Here's how the part is built. I have some questions about the finished solid (model axes, mm). Face numbers are marked on the shaded views. Round coordinates to 2 decimals unless told otherwise and drop trailing zeros. Loops run counter-clockwise (first coordinate to the right, second up) from the corner with the lowest first, then second, coordinate; pieces in that order, holes last. Notation, with made-up numbers: M -28,20 L -6,20 A20 ccw -6,48 Z; hole C 88.5,64 d3. An arc over 180 degrees is marked long. Answer as a JSON object with one key per item and string values.
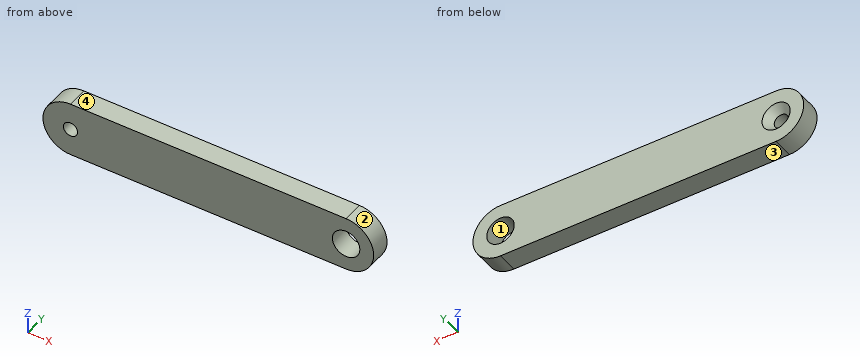
from build123d import *

# Parameters (mm, degrees)
BOSS_EXTRUDE2_DEPTH                               = 4.7625
SKETCH2_R                                         = 3.1623
CUT_EXTRUDE1_DEPTH                                = 5.7625
CSK_FOR_4_FLAT_HEAD_SOCKET_CAP_SCREW1_D           = 3.2639
CSK_FOR_4_FLAT_HEAD_SOCKET_CAP_SCREW1_CSINK_D     = 6.477
CSK_FOR_4_FLAT_HEAD_SOCKET_CAP_SCREW1_CSINK_ANGLE = 82


with BuildPart() as part:
    # Sketch1 → Boss-Extrude2 (new body)
    with BuildSketch(Plane(origin=(0, 0, 0), x_dir=(1, 0, 0), z_dir=(0, 1, 0))):
        with BuildLine():
            Line((-63.5, 6.35), (0, 6.35))
            ThreePointArc((0, 6.35), (6.35, 0), (0, -6.35))
            Line((0, -6.35), (-63.5, -6.35))
            ThreePointArc((-63.5, -6.35), (-69.85, 0), (-63.5, 6.35))
        make_face()
    extrude(amount=BOSS_EXTRUDE2_DEPTH)

    # Sketch2 → Cut-Extrude1 (cut, through all)
    with BuildSketch(Plane(origin=(0, 4.7625, 0), x_dir=(1, 0, 0), z_dir=(0, 1, 0))):
        Circle(SKETCH2_R)
    extrude(amount=-CUT_EXTRUDE1_DEPTH, mode=Mode.SUBTRACT)

    # CSK for #4 Flat Head Socket Cap Screw1 (through all)
    with Locations(Plane(origin=(0, 4.7625, 0), x_dir=(1, 0, 0), z_dir=(0, 1, 0))):
        with Locations((-63.5, 0)):
            CounterSinkHole(CSK_FOR_4_FLAT_HEAD_SOCKET_CAP_SCREW1_D / 2, CSK_FOR_4_FLAT_HEAD_SOCKET_CAP_SCREW1_CSINK_D / 2, counter_sink_angle=CSK_FOR_4_FLAT_HEAD_SOCKET_CAP_SCREW1_CSINK_ANGLE)


solid = part.part
Item 1: I want a section at A-A on z = 0. List the corners of the cut face in (x, y) for me, plus the area to 3 significant figures.
Solution:
{"outline": "M -69.85,0 L -65.13,0 L -65.13,2.91 L -66.74,4.76 L -69.85,4.76 Z; M -61.87,0 L -3.16,0 L -3.16,4.76 L -60.26,4.76 L -61.87,2.91 Z; M 3.16,0 L 6.35,0 L 6.35,4.76 L 3.16,4.76 Z", "area": "314 mm2"}
Item 2: If I drill on L1, parallel to X at y = 4.45, z = -2.25; L2, parallel to Z at x = -63.5, y = 1.1; L3, parallel to X at y = 3.05, z = 1, over which ranges is the centre line in solid material (lowest first)? Write a range as from..to.
Solution:
{"L1": "x = -69.44..-65.43, -61.57..-2.22, 2.22..5.94", "L2": "z = -6.35..-1.63, 1.63..6.35", "L3": "x = -69.77..-64.94, -62.06..-3, 3..6.27"}
Item 3: I want a section at C-C on z = -4.25. List the corners of the cut face in (x, y) for me, plus the area to 3 significant figures.
Solution:
{"outline": "M -68.22,0 L 4.72,0 L 4.72,4.76 L -68.22,4.76 Z", "area": "347 mm2"}
Item 4: For P1, Ø3, axis at x = -63.5, z = 0, coming from the -Y side; P2, Ø4, axis at x = -20.5, z = -2, coming from the -Y side, each with a flat end and sliding along its axis, tell me the tip position at first contact or that it passes through.
Solution:
{"P1": "passes through", "P2": "stops at y = 0"}
Item 5: I want a section at B-B on y = 2.2. List the corners of the cut face in (x, z) for me.
Solution:
{"outline": "M -63.5,-6.35 L 0,-6.35 A6.35 ccw 0,6.35 L -63.5,6.35 A6.35 ccw Z; hole C -63.5,0 d3.26; hole C 0,0 d6.32"}
Item 6: We'd pull the mould along Z, two halves only. Please class the marked faces 1, 2, 3 and 4: +Z half, -Z half, draft (parallel to the pull), parting line (faces both ways), or undercut.
Solution:
{"face 1": "undercut", "face 2": "parting line", "face 3": "-Z half", "face 4": "+Z half"}
